Source: CAD feature listing. Evaluate the final solid. Frame: model axes, mm. Give positions to 0.01 mm unless a question says otherwise; leave off trailing zeros. Order: outer loops, then holes, each group sorted by start corner. A loop starts at its lowest first (then second) coordinate and runs counter-clockwise, first axis right, second up. Notation, with made-up numbers: M 53,-38 L 105,-38 A15 ccw 105,-20 Z; hole C 7,-13 d1. An arc over 180 degrees is marked long. Answer as a JSON object with one key per item and string values. Group by question number.
1. Section query D-D (x = -12.7). Output: boundary loops of the cut face in (y, z) (3 decimals).
2. Section query A-A (y = -1.45). Output: boundary loops of the cut face in (x, z), plus the area to 3 significant figures.
3. Section query C-C (z = -50.8). Output: boundary loops of the cut face in (x, y) (3 decimals).
4. Pin query (flat end, axial travel): P1, Ø1, axis at x = 2.5, y = -0.5, coming from the +Z side; P2, Ø1.5, axis at x = -17.5, y = -1.5, coming from the +Z side; P3, Ø8, axis at x = 18.5, z = -30.5, coming from the +Y side. Return the tip coordinate at first contact, or that it passes through.
5. Section query B-B (x = 0). Output: boundary loops of the cut face in (y, z) (3 decimals), plus the area to 3 significant figures.
6. Material intervals for L1, parallel to Z at x = 0, y = -1.4; L2, parallel to X at y = -0.4, z = -53; L3, parallel to Z at x = -1, y = -2.7, sorted ascending. Write a range as [from, to].
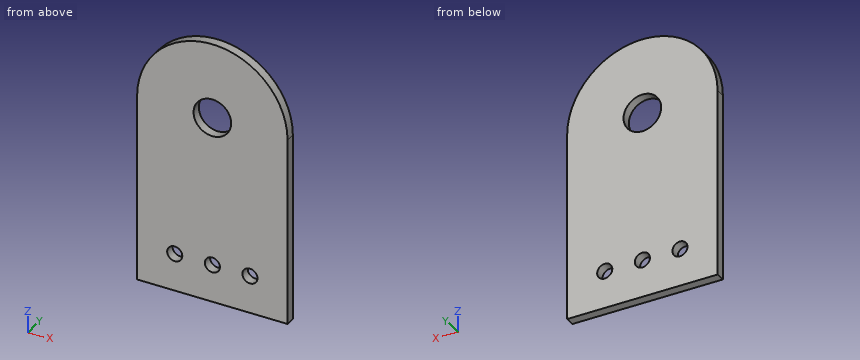
from build123d import *

# Parameters (mm, degrees)
F0_R     = 2.5527
F0_R_2   = 6.35
F1_DEPTH = 3.175


with BuildPart() as f1:
    # F0 (on Front) → F1 (new body)
    with BuildSketch(Plane.XZ):
        with BuildLine():
            Line((25.4, -63.5), (25.4, 0))
            ThreePointArc((25.4, 0), (0, 25.4), (-25.4, 0))
            Line((-25.4, 0), (-25.4, -63.5))
            Line((-25.4, -63.5), (25.4, -63.5))
        make_face()
        with Locations((-12.7, -50.8)):
            Circle(F0_R, mode=Mode.SUBTRACT)
        with Locations((0, -50.8)):
            Circle(F0_R, mode=Mode.SUBTRACT)
        with Locations((12.7, -50.8)):
            Circle(F0_R, mode=Mode.SUBTRACT)
        Circle(F0_R_2, mode=Mode.SUBTRACT)
    extrude(amount=F1_DEPTH)


solid = f1.part
Answer sheet:
{
 "1": {"outline": "M -3.175,-63.5 L 0,-63.5 L 0,-53.353 L -3.175,-53.353 Z; M -3.175,-48.247 L 0,-48.247 L 0,21.997 L -3.175,21.997 Z"},
 "2": {"outline": "M -25.4,-63.5 L 25.4,-63.5 L 25.4,0 A25.4 ccw -25.4,0 Z; hole C -12.7,-50.8 d5.11; hole C 0,0 d12.7; hole C 0,-50.8 d5.11; hole C 12.7,-50.8 d5.11", "area": "4,050 mm^2"},
 "3": {"outline": "M -25.4,-3.175 L -15.253,-3.175 L -15.253,0 L -25.4,0 Z; M -10.147,-3.175 L -2.553,-3.175 L -2.553,0 L -10.147,0 Z; M 2.553,-3.175 L 10.147,-3.175 L 10.147,0 L 2.553,0 Z; M 15.253,-3.175 L 25.4,-3.175 L 25.4,0 L 15.253,0 Z"},
 "4": {"P1": "z = 25.32", "P2": "z = 19.09", "P3": "y = 0"},
 "5": {"outline": "M -3.175,-63.5 L 0,-63.5 L 0,-53.353 L -3.175,-53.353 Z; M -3.175,-48.247 L 0,-48.247 L 0,-6.35 L -3.175,-6.35 Z; M -3.175,6.35 L 0,6.35 L 0,25.4 L -3.175,25.4 Z", "area": "226 mm^2"},
 "6": {"L1": "[-63.5, -53.35], [-48.25, -6.35], [6.35, 25.4]", "L2": "[-25.4, -13.99], [-11.41, -1.29], [1.29, 11.41], [13.99, 25.4]", "L3": "[-63.5, -53.15], [-48.45, -6.27], [6.27, 25.38]"}
}
